Source: three-view drawing plus pictorial views. Frame: mm from the lowest corner of the part. Round coordinates to 2 decimals unless told otherwise and drop trailing zeros. Loops run counter-clockwise (first coordinate to the right, second up) from the corner with the lowest first, then second, coordinate; pieces in that order, holes last. Notation, with made-up numbers: M 49,6.5 L 76,6.5 A20 cw 76,30.5 Z; hole C -36.75,-10 d5. An arc over 180 degrees is marked long. Return JSON: item names as keys, results as strings. Group by question number.
1) Section D-D (y = 0.5). Count the separate pieces of the cut face and the enclosed holes in it, plus the area to 3 significant figures.
2) Section A-A (z = 42). Output: boundary loops of the cut face in (x, y).
3) Material intervals for line 1 (X direction, y = 0.9, z = 79.5); line 2 (Z direction, x = 91.5, y = 2.5); line 3 (Z direction, x = 100, y = 1.55) (3 decimals), sorted ascending. Write a range as from..to.
4) Section C-C (x = 114). Output: boundary loops of the cut face in (y, z).
5) Contact query for flat-ended pins moving along their axis: P1, Ø5.5, axis at x = 35.9, z = 4.5, coming from the +Y side; P2, Ø1.5, axis at x = 100, y = 1.5, coming from the -Z side. Output: stop coordinate, or through.
6) Section B-B (x = 35.9). Output: boundary loops of the cut face in (y, z).
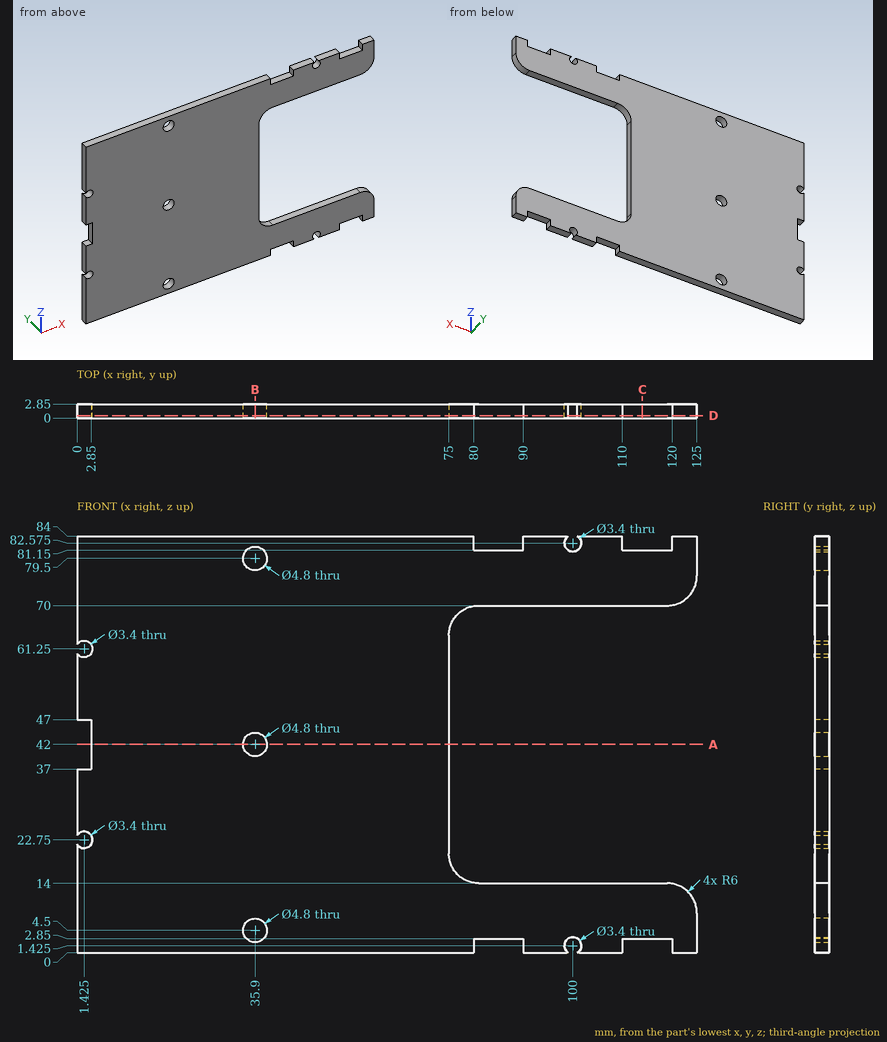
Returned:
{
 "1": {"separate pieces": "1", "enclosed holes": "3", "area": "7,470 mm^2"},
 "2": {"outline": "M 2.85,0 L 33.5,0 L 33.5,2.85 L 2.85,2.85 Z; M 38.3,0 L 75,0 L 75,2.85 L 38.3,2.85 Z"},
 "3": {"line 1": "x = 0..33.5, 38.3..125", "line 2": "z = 0..14, 70..84", "line 3": "z = 3.125..14, 70..80.875"},
 "4": {"outline": "M 0,2.85 L 2.85,2.85 L 2.85,14 L 0,14 Z; M 0,70 L 2.85,70 L 2.85,81.15 L 0,81.15 Z"},
 "5": {"P1": "stops at y = 2.85", "P2": "stops at z = 2.95"},
 "6": {"outline": "M 0,0 L 2.85,0 L 2.85,2.1 L 0,2.1 Z; M 0,6.9 L 2.85,6.9 L 2.85,39.6 L 0,39.6 Z; M 0,44.4 L 2.85,44.4 L 2.85,77.1 L 0,77.1 Z; M 0,81.9 L 2.85,81.9 L 2.85,84 L 0,84 Z"}
}
